Print and shaded views of the part. All mm, measured from the part's lowest x, y and z. Round coordinates to 2 decimals unless told otherwise and drop trailing zeros. Write each loop counter-clockwise with the first axis right and the second up, starting at its lowest first coordinate (ties: lowest second). Pieces come first, ordered by that corner, then holes. Notation, with made-up numbers: (28, -32) - (71, -32) arc R30 ccw to (71, -1) - close; hole circle Ø4 at (16.5, -12). An arc over 180 degrees is marked (long way). One line per item, written item: value.
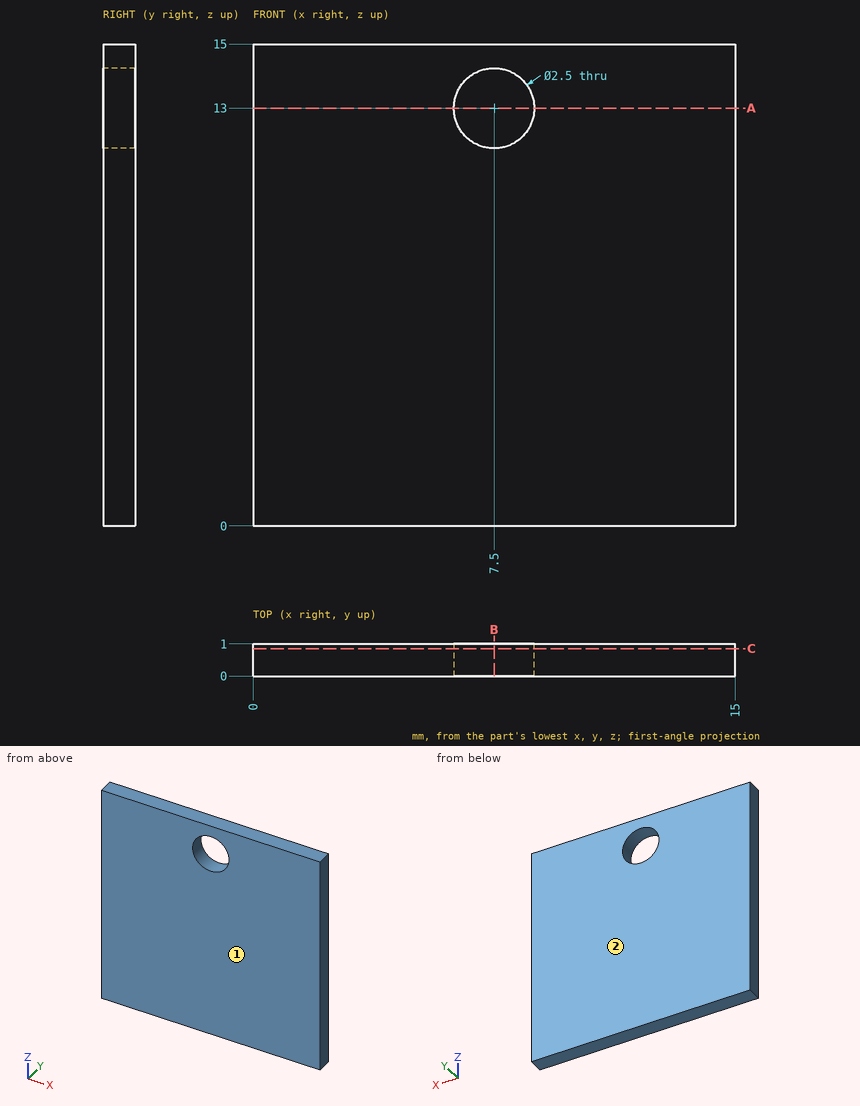
1. Band-saw the part on B-B on x = 7.5. Write the cut outline in (y, z), plus the area to 3 significant figures.
Report:
outline: (0, 0) - (1, 0) - (1, 11.75) - (0, 11.75) - close; (0, 14.25) - (1, 14.25) - (1, 15) - (0, 15) - close
area: 12.5 mm²
2. Mould opens along Y. For the marked faces 1 and 2 say: released by +Y, released by -Y, zero draft, split by the parting line, or undercut.
Report:
face 1: released by -Y
face 2: released by +Y
3. Band-saw the part on C-C on y = 0.85. Write the cut outline in (x, z), plus the area to 3 significant figures.
Report:
outline: (0, 0) - (15, 0) - (15, 15) - (0, 15) - close; hole circle Ø2.5 at (7.5, 13)
area: 220 mm²
4. Wall check: probe 1 along X at (y, z) = (0.5, 13); probe 2 along Z at (x, y) = (7.5, 0.6); probe 3 along X at (y, z) = (0.1, 12.25). Give the ranges that are in metal, low to high. Write a range as [from, to].
Report:
probe 1: [0, 6.25], [8.75, 15]
probe 2: [0, 11.75], [14.25, 15]
probe 3: [0, 6.5], [8.5, 15]
5. Band-saw the part on A-A on z = 13. Write the cut outline in (x, y), plus the area to 3 significant figures.
Report:
outline: (0, 0) - (6.25, 0) - (6.25, 1) - (0, 1) - close; (8.75, 0) - (15, 0) - (15, 1) - (8.75, 1) - close
area: 12.5 mm²
